For this review, use the dimensioned drawing (mm, ordinates from the lowest corner) and the shaded views. A direction names the side the tool comes from. Coordinates: 2 decimals unless noted, no trailing zeros. Write each loop counter-clockwise with the first axis right and the second up, starting at its lowest first coordinate (ties: lowest second). Pieces come first, ordered by that corner, then holes.
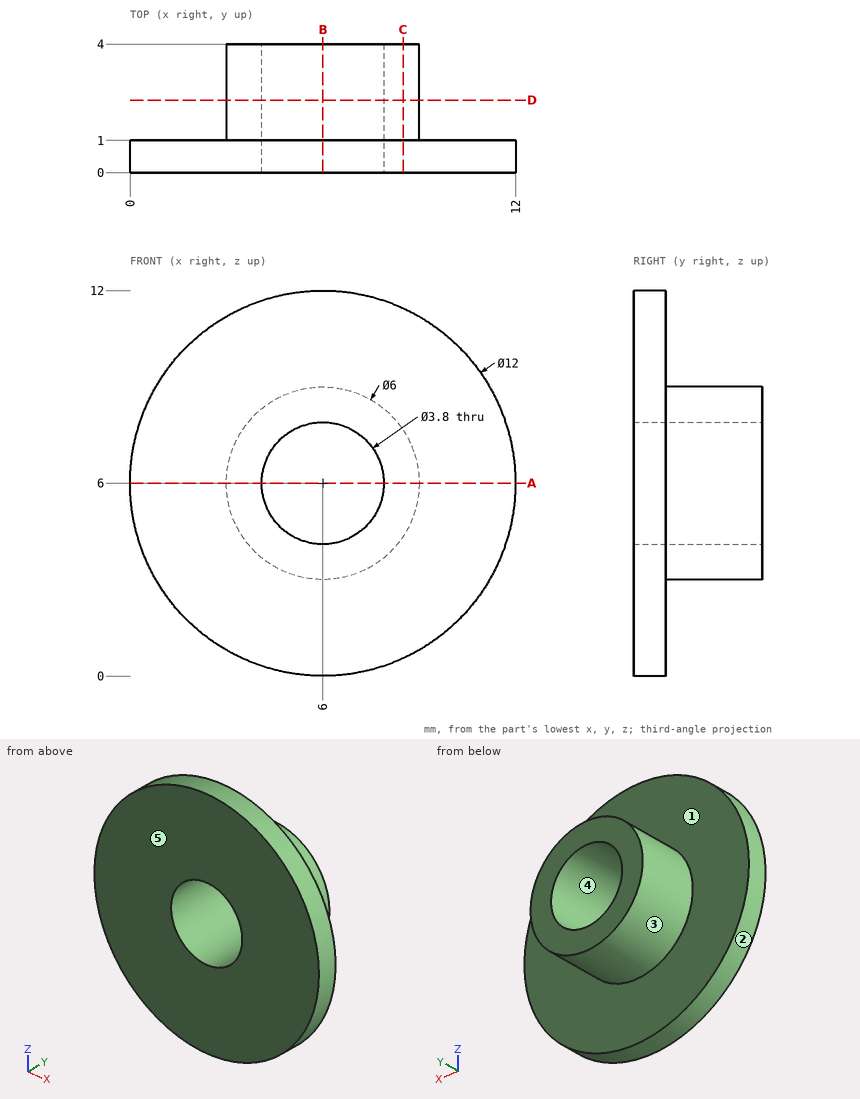
(1) Consider section C-C (x = 8.5). Give the boundary of the cut face in (y, z), plus the area to 3 significant figures.
(2) Consider section D-D (y = 2.25). Give the boundary of the cut face in (x, z).
(3) Consider section B-B (x = 6). Give the boundary of the cut face in (y, z).
(4) Insertion check: pin 1 Ø1 at (x, y) = (3, 3.5) entering from +Z. The pin has a flat end and moves straight along its axis. Give the tip position at first contact, or say it passes through.
(5) Wall thickness on line 1 (Z direction, x = 6, y = 3.2); line 2 (Y direction, x = 9.5, z = 2.5): over which ranges is each line inside the solid? List them lowest first.
(6) Consider section A-A (z = 6). Give the boundary of the cut face in (x, y).
(7) For the marked faces 1 and 2, list the 3-axis set-ups (+Z, -Z, +X, -X, +Y, -Y) from which the entire face can be reached by the end or side of a thin tool; tool diameter is ignored.
(8) Mouldability with a two-part tool opening along Z and no side actions: class the marked faces 3, 4 and 5 as +Z half, -Z half, draft (parallel to the pull), parting line (faces both ways), or undercut.
Results:
1. outline: (0, 0.55) - (1, 0.55) - (1, 4.34) - (4, 4.34) - (4, 7.66) - (1, 7.66) - (1, 11.45) - (0, 11.45) - close
1. area: 20.9 mm2
2. outline: circle Ø6 at (6, 6); hole circle Ø3.8 at (6, 6)
3. outline: (0, 0) - (1, 0) - (1, 3) - (4, 3) - (4, 4.1) - (0, 4.1) - close; (0, 7.9) - (4, 7.9) - (4, 9) - (1, 9) - (1, 12) - (0, 12) - close
4. pin 1: stops at z = 7.66
5. line 1: z = 3 to 4.1, 7.9 to 9
5. line 2: y = 0 to 1
6. outline: (0, 0) - (4.1, 0) - (4.1, 4) - (3, 4) - (3, 1) - (0, 1) - close; (7.9, 0) - (12, 0) - (12, 1) - (9, 1) - (9, 4) - (7.9, 4) - close
7. face 1: +Y
7. face 2: +Y, -Y
8. face 3: parting line
8. face 4: undercut
8. face 5: draft
